Source: CAD feature listing. Evaluate the final solid. Frame: model axes, mm. Face numbers are marked on the shaded views. A direction names the side the tool comes from. Give positions to 0.01 mm unless a question says otherwise; leave off trailing zeros. Order: outer loops, then holes, each group sorted by start corner. A loop starts at its lowest first (then second) coordinate and runs counter-clockwise, first axis right, second up. Notation, with made-up numbers: M 9,-3 L 32,-3 A19 cw 32,18 Z; hole C 6.5,32 d5. An arc over 180 degrees is marked long. Use CSV: the item, a comma, the result in double quotes. Start each with the question number.
Item 1: First-contact query: pin 1 (8 mm diameter, centred on y = 20, z = 5, fed in from -X); pin 2 (10.5 mm diameter, centred on y = 10.5, z = 11.5, fed in from +X); pin 3 (6 mm diameter, centred on x = -4.5, z = 6.5, fed in from +Y). Flat tips, straight axial feed; report the tip coordinate or a pass-through.
Item 2: Section query A-A on z = 25.5. Return loops of the section in (x, y).
Item 3: Ray query, probe 1 along X at (y, z) = (0.7, -25.5); probe 2 along Y at (x, z) = (0, -1.85); probe 3 along Y at (x, z) = (-3, 4). Return the intervals inside material, ascending. Write a range as from..to.
Item 4: Section query C-C on x = -7.5. Return loops of the section in (y, z).
Item 5: Access query for the marked faces 1, 2 and 3. Directions: +Z, -Z, +X, -X, +Y, -Y. A direction counts if a zero-diameter tool reaches every point of the face in a straight line with its end or side. Return the directions, or none.
Item 6: Section query B-B on x = -1.5. Return loops of the section in (y, z).
Item 7: Section query D-D on z = -11. Return loops of the section in (x, y), and give its area (3 significant figures).
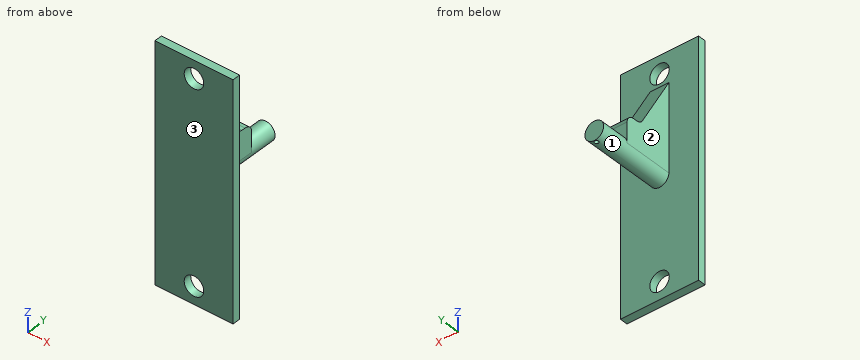
from build123d import *

# Parameters (mm, degrees)
SKETCH1_W           = 20
SKETCH1_H           = 60
BOSS_EXTRUDE1_DEPTH = 2
SKETCH2_R           = 2.5
CUT_EXTRUDE1_DEPTH  = 32.685959036
SKETCH3_R           = 2.4
BOSS_EXTRUDE2_DEPTH = 20
BOSS_EXTRUDE7_DEPTH = 4.8
CUT_EXTRUDE2_START  = -1
SKETCH5_R           = 0.5
CUT_EXTRUDE2_DEPTH  = 2


with BuildPart() as part:
    # Sketch1 → Boss-Extrude1 (new body)
    with BuildSketch(Plane(origin=(0, 0, 0), x_dir=(1, 0, 0), z_dir=(0, 1, 0))):
        Rectangle(SKETCH1_W, SKETCH1_H)
    extrude(amount=BOSS_EXTRUDE1_DEPTH)

    # Sketch2 → Cut-Extrude1 (cut, through all)
    with BuildSketch(Plane(origin=(0, 2, 0), x_dir=(1, 0, 0), z_dir=(0, 1, 0))):
        with Locations(Location((0, 25.5, 0), (0, 0, 270))):
            Circle(SKETCH2_R)
        with Locations(Location((0, -25.5, 0), (0, 0, 90))):
            Circle(SKETCH2_R)
    extrude(amount=-CUT_EXTRUDE1_DEPTH, mode=Mode.SUBTRACT)

    # Sketch3 → Boss-Extrude2 (add)
    with BuildSketch(Plane(origin=(0, 2, 0), x_dir=(1, 0, 0), z_dir=(0, 1, 0))):
        with Locations(Location((0, 0, 0), (0, 0, 270))):
            Circle(SKETCH3_R)
    extrude(amount=BOSS_EXTRUDE2_DEPTH)

    # Sketch4 → Boss-Extrude7 (add)
    with BuildSketch(Plane.ZY.offset(2.4)):
        with BuildLine():
            Line((8.130845775, 10.120752848), (22.196402304, 2))
            Line((22.196402304, 2), (0, 2))
            Line((0, 2), (0, 14.815098845))
            Line((0, 14.815098845), (5.130845775, 14.815098845))
            ThreePointArc((5.130845775, 14.815098845), (6.545059338, 14.229312408), (7.130845775, 12.815098845))
            Line((7.130845775, 12.815098845), (7.130845775, 11.852803656))
            ThreePointArc((7.130845775, 11.852803656), (7.398794968, 10.852803656), (8.130845775, 10.120752848))
        make_face()
    extrude(amount=-BOSS_EXTRUDE7_DEPTH)

    # Sketch5 → Cut-Extrude2 (cut)
    with BuildSketch(Plane.XY.offset(CUT_EXTRUDE2_START)):
        with Locations((0, 21.3)):
            Circle(SKETCH5_R)
    extrude(amount=-CUT_EXTRUDE2_DEPTH, mode=Mode.SUBTRACT)


solid = part.part
Verdict:
1,pin 1,"x = -2.18"
1,pin 2,"x = 2.4"
1,pin 3,"y = 14.82"
2,outline,"M -10,0 L -2.5,0 L -2.5,2 L -10,2 Z; M 2.5,0 L 10,0 L 10,2 L 2.5,2 Z"
3,probe 1,"-10..-2.5, 2.5..10"
3,probe 2,"0..20.8, 21.8..22"
3,probe 3,"0..2"
4,outline,"M 0,-30 L 2,-30 L 2,30 L 0,30 Z"
5,face 1,"+Y"
5,face 2,"+Z, -Z, -X, +Y"
5,face 3,"+Z, -Z, +X, -X, -Y"
6,outline,"M 0,-30 L 2,-30 L 2,-27.5 L 0,-27.5 Z; M 0,-23.5 L 2,-23.5 L 2,-1.87 L 22,-1.87 L 22,1.87 L 14.82,1.87 L 14.82,5.13 A2 ccw 12.82,7.13 L 11.85,7.13 A2 cw 10.12,8.13 L 2,22.2 L 2,23.5 L 0,23.5 Z; M 0,27.5 L 2,27.5 L 2,30 L 0,30 Z"
7,outline,"M -10,0 L 10,0 L 10,2 L -10,2 Z"
7,area,"40.0 mm2"
